Autodesk Inventor part; units mm, degrees
ref_plane "YZ Plane" through (0, 0, 0) normal (1, 0, 0) x (0, 1, 0)
ref_plane "XZ Plane" through (0, 0, 0) normal (0, 1, 0) x (-1, 0, 0)
ref_plane "XY Plane" through (0, 0, 0) normal (0, 0, 1) x (1, 0, 0)
sketch "Sketch1" plane through (0, 0, 0) normal (0, 0, 1) x (1, 0, 0)
  line L0 (0, 0) -> (0, 87.5)
  line L1 (0, 87.5) -> (43.6046, 111.967)
  line L2 (0, 0) -> (50, 0)
  line L3 (50, 0) -> (93.217, 25.1454)
  circle A0 centre (68.0717, 68.3624) radius 50 construction
  arc A1 (93.217, 25.1454) -> (43.6046, 111.967) centre (68.0717, 68.3624) ccw
  dimension "d0" = 87.5
  dimension "d1" = 50
  dimension "d2" = 50
  dimension "d3" = 50
  dimension "d4" = 100
extrude "Extrusion1" add sketch "Sketch1" along normal blind 50
sketch "Sketch2" plane through (0, 0, 50) normal (0, 0, 1) x (1, 0, 0)
  line L0 (0, 0) -> (50, 0)
  line L1 (50, 0) -> (93.217, 25.1454)
  arc A0 (93.217, 25.1454) -> (43.6046, 111.967) centre (68.0717, 68.3624) ccw
  line L2 (43.6046, 111.967) -> (0, 87.5)
  line L3 (0, 81.7667) -> (46.0513, 107.6066)
  arc A1 (90.7025, 29.4671) -> (46.0513, 107.6066) centre (68.0717, 68.3624) ccw
  line L4 (90.7025, 29.4671) -> (48.6512, 5)
  line L5 (48.6512, 5) -> (0, 5)
  line L6 (0, 87.5) -> (0, 0)
  line L7 (0, 5) -> (0, 81.7667)
  dimension "d7" = 5
extrude "Extrusion2" cut sketch "Sketch2" against normal blind 45 contours L6 L3 A1 L4 L5
sketch "Sketch3" plane through (0, 0, 0) normal (-1, 0, 0) x (0, 0, 1)
  line L0 (0, 87.5) -> (50, 87.5)
  line L1 (50, 113.3624) -> (50, 29.4671)
  line L2 (0, 87.5) -> (50, 87.5)
  line L3 (50, 87.5) -> (50, 72.5)
  line L4 (50, 72.5) -> (0, 72.5)
  line L5 (0, 72.5) -> (0, 87.5)
  point P0 (0, 0)
  point P1 (50, 107.6066)
  dimension "d10" = 15
extrude "Extrusion3" add sketch "Sketch3" against normal blind 5
sketch "Sketch4" plane through (0, 0, 0) normal (-1, 0, 0) x (0, 0, 1)
  line L0 (0, 87.5) -> (0, 111.967)
  line L1 (0, 87.5) -> (15, 87.5)
  line L2 (15, 87.5) -> (15, 32.5)
  line L3 (15, 32.5) -> (0, 32.5)
  line L4 (0, 32.5) -> (0, 87.5)
  line L5 (0, 0) -> (50, 0)
  dimension "d13" = 15
  dimension "d14" = 32.5
extrude "Extrusion4" add sketch "Sketch4" against normal blind 5
sketch "Sketch6" plane through (0, 0, 5) normal (0, 0, 1) x (1, 0, 0)
  circle A0 centre (21.5, 30) radius 20
  line L0 (48.6512, 5) -> (0, 5)
  line L1 (0, 5) -> (0, 32.5)
  circle A1 centre (21.5, 30) radius 5
  point P0 (0, 0)
  dimension "d22" = 40
  dimension "d37" = 25
  dimension "d38" = 21.5
  dimension "d39" = 10
sketch "Sketch7" plane through (0, 0, 5) normal (0, 0, 1) x (1, 0, 0)
  arc A0 (93.217, 25.1454) -> (43.6046, 111.967) centre (68.0717, 68.3624) ccw
  circle A1 centre (68.0717, 68.3624) radius 6.25
  circle A2 centre (68.0717, 68.3624) radius 21.25
  point P0 (0, 0)
  dimension "d25" = 12.5
  dimension "d28" = 15
extrude "Extrusion8" add sketch "Sketch7" along normal blind 10
sketch "Sketch8" plane through (68.0717, 68.3624, 5) normal (0, 0, 1) x (1, 0, 0)
  circle A0 centre (0, 0) radius 6.25
  circle A1 centre (0, 0) radius 6.25
  point P0 (-68.0717, -68.3624)
extrude "Extrusion9" cut sketch "Sketch8" against normal through all
sketch "Sketch9" plane through (0, 0, 0) normal (0, 0, -1) x (-1, 0, 0)
  circle A0 centre (-68.0717, 68.3624) radius 21.25
  circle A1 centre (-68.0717, 68.3624) radius 21.25
  point P0 (0, 0)
extrude "Extrusion10" add sketch "Sketch9" along normal blind 5
sketch "Sketch10" plane through (0, 0, 50) normal (0, 0, 1) x (1, 0, 0)
  arc A0 (93.217, 25.1454) -> (43.6046, 111.967) centre (68.0717, 68.3624) ccw
  circle A1 centre (68.0717, 68.3624) radius 50
  line L0 (18.0717, 68.3624) -> (18.0717, 97.6402)
  line L1 (0, 87.5) -> (43.6046, 111.967)
  line L2 (43.6046, 111.967) -> (18.0717, 97.6402)
  line L3 (68.0717, 18.3624) -> (81.5592, 18.3624)
  line L4 (50, 0) -> (93.217, 25.1454)
  line L5 (81.5592, 18.3624) -> (93.217, 25.1454)
  point P0 (0, 0)
extrude "Extrusion11" cut sketch "Sketch10" against normal blind 10
extrude "Extrusion12" add sketch "Sketch6" along normal blind 10
sketch "Sketch11" plane through (0, 0, 5) normal (0, 0, 1) x (1, 0, 0)
  circle A0 centre (15, 78.7167) radius 10
  circle A1 centre (15, 78.7167) radius 2.5
  line L0 (5, 84.5722) -> (18.0717, 91.9069)
  line L1 (5, 84.5722) -> (5, 72.5)
  point P0 (0, 0)
  dimension "d42" = 20
  dimension "d43" = 5
extrude "Extrusion13" add sketch "Sketch11" along normal blind 45 contours A0
sketch "Sketch12" plane through (0, 0, 5) normal (0, 0, 1) x (1, 0, 0)
  line L0 (1.6569, 32.5) -> (0, 32.5)
  line L1 (0, 32.5) -> (5, 32.5)
  line L2 (5, 32.5) -> (5, 5)
  line L3 (5, 5) -> (0, 5)
  line L4 (0, 5) -> (0, 32.5)
  point P0 (0, 0)
  dimension "d46" = 5
extrude "Extrusion14" cut sketch "Sketch12" along normal through all
sketch "Sketch13" plane through (68.0717, 68.3624, -5) normal (0, 0, -1) x (-1, 0, 0)
  circle A0 centre (0, 0) radius 21.25
  circle A1 centre (46.5717, -38.3624) radius 5
  circle A2 centre (46.5717, -38.3624) radius 2.5
  circle A3 centre (0, 0) radius 6.25
  circle A4 centre (0, 0) radius 2.5
  point P0 (68.0717, -68.3624)
  dimension "d49" = 5
  dimension "d50" = 5
extrude "Extrusion15" cut sketch "Sketch13" against normal through all contours A2 | A4
properties part number "BA005" material "ABS Plastic"
Geometry: final body of the model. Coordinates: model frame, mm. A direction names the side the tool comes from. Coordinates: 2 decimals unless noted, no trailing zeros. Order: outer loops, then holes, each group sorted by start corner. A loop starts at its lowest first (then second) coordinate and runs counter-clockwise, first axis right, second up.
1) Section B-B (x = 21.5). Return loops of the section in (y, z).
Result sheet:
outline: (0, 0) - (27.5, 0) - (27.5, 5) - (25, 5) - (25, 15) - (10, 15) - (10, 5) - (5, 5) - (5, 50) - (0, 50) - close; (32.5, 0) - (99.56, 0) - (99.56, 40) - (93.83, 40) - (93.83, 5) - (86.32, 5) - (86.32, 50) - (71.12, 50) - (71.12, 5) - (50, 5) - (50, 15) - (35, 15) - (35, 5) - (32.5, 5) - close
2) First-contact query: P1, Ø18.5, axis at y = 62, z = 32, coming from the +X side; P2, Ø12.5, axis at x = 18, y = 52, coming from the +Z side; P3, Ø10, axis at x = 73, z = 43.5, coming from the -Y side; P4, Ø5, axis at x = 44, z = 36, coming from the +Y side. Flat tips, straight axial feed; report the tip coordinate or a pass-through.
Result sheet:
P1: stops at x = 118.07
P2: stops at z = 15
P3: stops at y = 10.47
P4: stops at y = 113.47
3) Section D-D (y = 59.5). Return loops of the section in (x, z), then the cut area to 3 significant figures.
Result sheet:
outline: (0, 0) - (48.76, 0) - (48.76, -5) - (87.39, -5) - (87.39, 0) - (117.28, 0) - (117.28, 40) - (112.19, 40) - (112.19, 5) - (87.39, 5) - (87.39, 15) - (48.76, 15) - (48.76, 5) - (5, 5) - (5, 15) - (0, 15) - close
area: 1,390 mm2
4) Set-up query: faces 1 (the flat face through (16, 35, 15)), 2 (the flat face through (69.971, 17.405, 27.815)), 3 (the flat face through (18.072, 95, 45)), 4 (the cylindrical face through (47.803, 61.979, -2.465)). Return all of +Z, -Z, +X, -X, +Y, -Y with unobstructed straight access to the full face (end or side cutting, diameter ignored); none if empty.
Result sheet:
face 1: +Z, -X
face 2: +Z
face 3: +Z, +X, +Y
face 4: -Z
5) Draft query along Z for faces 5 (the flat face through (45, 60, 0)), 6 (the flat face through (77, 18.362, 45)), 7 (the flat face through (6, 84, 5)). Return one class per face: released by +Z, released by -Z, zero draft, split by the parting line, or undercut.
Result sheet:
face 5: released by -Z
face 6: zero draft
face 7: released by +Z
6) Ray query, probe 1 along Y at (x, z) = (21.5, 11.5); probe 2 along X at (y, z) = (46.5, 8.5); probe 3 along Z at (x, y) = (91, 77.5). Return the intervals inside material, ascending.
Result sheet:
probe 1: y = 0 to 5, 10 to 25, 35 to 50, 71.12 to 86.32, 93.83 to 99.56
probe 2: x = 0 to 5, 10.2 to 32.8, 107.4 to 113.04
probe 3: z = 0 to 5
